The figure shows three views and two pictorial views of one solid part (mm, origin at its lowest corner). Answer the questions. A direction names the side the tool comes from. Coordinates: 2 decimals unless noted, no trailing zeros. Order: outer loops, then holes, each group sorted by start corner. A loop starts at its lowest first (then second) coordinate and runs counter-clockwise, first axis right, second up. Notation, with made-up numbers: (-37.5, -16) -> (-16.5, -16) arc R30 cw to (-16.5, 17) -> close; hole circle Ø2 at (0, -16.5). An arc over 180 degrees is marked (long way). Write item = value, one per line. Start each with the question number.
Q1. For a pull along X with two mould halves and no side action, classify the marked faces 1, 2 and 3 as +X half, -X half, draft (parallel to the pull), parting line (faces both ways), or undercut.
Q2. The part is cut by section C-C, the plane x = 21.25. Determine the outline of the cut face in (y, z), plus the area to 3 significant figures.
Q3. The part is cut by section B-B, the plane z = 21.5. Determine the outline of the cut face in (x, y), plus the area to 3 significant figures.
Q4. Which of the six approach directions +Z, -Z, +X, -X, +Y, -Y give full straight-line access (tool end or side, diameter ignored) to the marked faces 4 and 5?
Q5. Flat-ended cylindrical pins translate along their axes: pin 1 (10 mm diameter, centred on x = 16.5, y = 11, fed in from +Z); pin 2 (1 mm diameter, centred on x = 22.5, z = 31.5, fed in from +Y). Find the tip coordinate at first contact, or state that the pin passes through.
Q6. Straight lines are drawn through the part: L1, parallel to X at y = 17.25, z = 30; L2, parallel to Z at x = 7.75, y = 15; L3, parallel to Y at x = 17.25, z = 29. For each, find the intervals that lie inside material, in ascending order. Write a range as from..to.
Q7. The part is cut by section A-A, the plane y = 13.5. Determine the outline of the cut face in (x, z), plus the area to 3 significant figures.
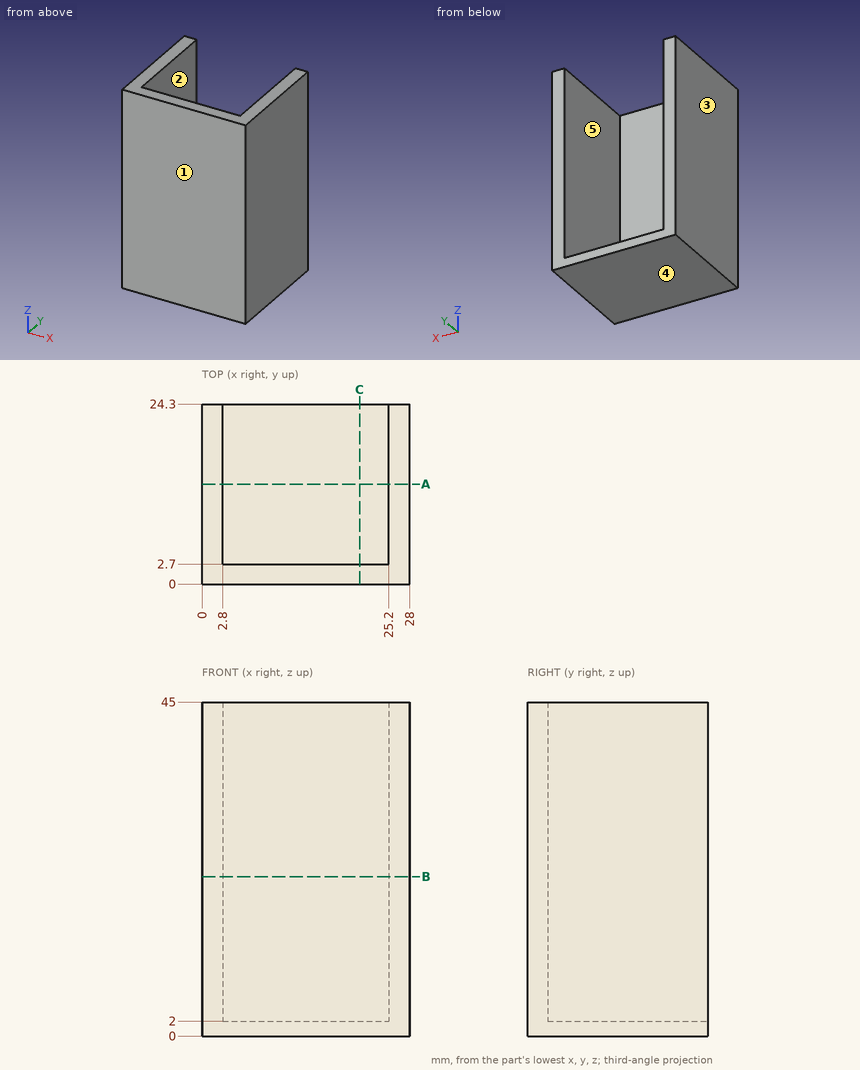
Model answer:
q1.face_1 = draft
q1.face_2 = undercut
q1.face_3 = -X half
q2.outline = (0, 0) -> (24.3, 0) -> (24.3, 2) -> (2.7, 2) -> (2.7, 45) -> (0, 45) -> close
q2.area = 165 mm2
q3.outline = (0, 0) -> (28, 0) -> (28, 24.3) -> (25.2, 24.3) -> (25.2, 2.7) -> (2.8, 2.7) -> (2.8, 24.3) -> (0, 24.3) -> close
q3.area = 197 mm2
q4.face_4 = -Z, +X, -X, +Y, -Y
q4.face_5 = +Z, +Y
q5.pin_1 = 2
q5.pin_2 = 2.7
q6.L1 = 0..2.8, 25.2..28
q6.L2 = 0..2
q6.L3 = 0..2.7
q7.outline = (0, 0) -> (28, 0) -> (28, 45) -> (25.2, 45) -> (25.2, 2) -> (2.8, 2) -> (2.8, 45) -> (0, 45) -> close
q7.area = 297 mm2
